Design review of the part shown in the three views and the two pictorial views. Dimensions are in mm from the part's minimum x, y and z. A direction names the side the tool comes from. Give positions to 0.01 mm unless a question says otherwise; leave off trailing zeros. Order: outer loops, then holes, each group sorted by start corner. A loop starts at its lowest first (then second) coordinate and runs counter-clockwise, first axis right, second up. Notation, with made-up numbers: M -26.75,39 L -2.75,39 A16 ccw -2.75,63 Z; hole C 41.5,-34 d10. An arc over 180 degrees is marked long. Answer as a JSON object with one key per item and string values.
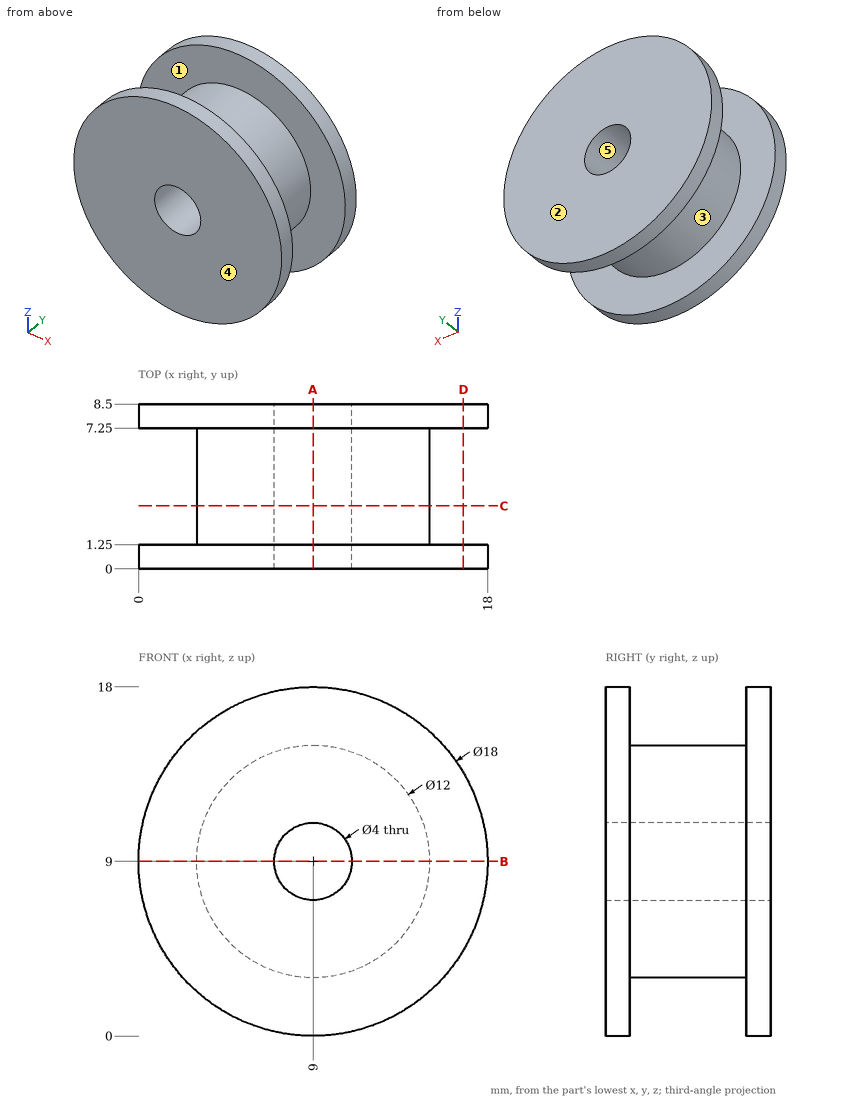
(1) To check wall thickness, follow L1, parallel to Y at x = 3, z = 14.25; L2, parallel to X at y = 6.25, z = 9; L3, parallel to Z at x = 8.75, y = 8. State the ranges of each line that lie inside material, in increasing order. Write a range as from..to.
Checked values:
{"L1": "y = 0..1.25, 7.25..8.5", "L2": "x = 3..7, 11..15", "L3": "z = 0..7.02, 10.98..18"}
(2) Draft analysis for pull direction X (two halves, no side actions). For the marked faces 3, 4 and 5, state which applies: +X half, -X half, draft (parallel to the pull), parting line (faces both ways), or undercut.
Checked values:
{"face 3": "parting line", "face 4": "draft", "face 5": "undercut"}
(3) Tool access review of the marked faces 1 and 2: name each direction out of +Z, -Z, +X, -X, +Y, -Y from which nothing blocks a thin tool from reaching the whole face with its end or side.
Checked values:
{"face 1": "none", "face 2": "+Z, -Z, +X, -X, +Y"}
(4) Insertion check: pin 1 (9 mm diameter, centred on x = 8, z = 11.5, fed in from -Y); pin 2 (3 mm diameter, centred on x = 3, y = 6, fed in from +Z); pin 3 (1 mm diameter, centred on y = 6.5, z = 4, fed in from +X); pin 4 (1 mm diameter, centred on x = 7, y = 3, fed in from +Z). Each pin has a flat end and moves straight along its axis. Give the tip position at first contact, or say it passes through.
Checked values:
{"pin 1": "stops at y = 0", "pin 2": "stops at z = 16.37", "pin 3": "stops at x = 12.97", "pin 4": "stops at z = 14.81"}
(5) We need section C-C (y = 3.25). Write out the cut boundary in (x, z).
Checked values:
{"outline": "C 9,9 d12; hole C 9,9 d4"}
(6) We need section A-A (x = 9). Write out the cut boundary in (y, z).
Checked values:
{"outline": "M 0,0 L 1.25,0 L 1.25,3 L 7.25,3 L 7.25,0 L 8.5,0 L 8.5,7 L 0,7 Z; M 0,11 L 8.5,11 L 8.5,18 L 7.25,18 L 7.25,15 L 1.25,15 L 1.25,18 L 0,18 Z"}
(7) We need section D-D (x = 16.75). Write out the cut boundary in (y, z), plus the area to 3 significant figures.
Checked values:
{"outline": "M 0,4.42 L 1.25,4.42 L 1.25,13.58 L 0,13.58 Z; M 7.25,4.42 L 8.5,4.42 L 8.5,13.58 L 7.25,13.58 Z", "area": "22.9 mm^2"}
(8) We need section B-B (z = 9). Write out the cut boundary in (x, y).
Checked values:
{"outline": "M 0,0 L 7,0 L 7,8.5 L 0,8.5 L 0,7.25 L 3,7.25 L 3,1.25 L 0,1.25 Z; M 11,0 L 18,0 L 18,1.25 L 15,1.25 L 15,7.25 L 18,7.25 L 18,8.5 L 11,8.5 Z"}
